Geometry: final body of the model. Coordinates: model frame, mm. Give positions to 0.01 mm unless a question says otherwise; leave off trailing zeros. Write each loop counter-clockwise with the first axis right and the second up, starting at its lowest first coordinate (ties: lowest second). Pieces come first, ordered by that corner, then holes. Notation, with made-up numbers: (43, 88) -> (87, 88) arc R26 ccw to (87, 113) -> close; hole circle Ø9 at (-21, 86.25). An arc over 180 degrees is marked (long way). Answer as a JSON object with one key per item and string values. Group by question number.
(1) Material intervals for probe 1 along Y at (x, z) = (0, 0); probe 2 along X at (y, z) = (0.5, 35); probe 3 along X at (y, z) = (3.5, 13.5), sorted ascending.
(2) Section query A-A on x = 0. Output: boundary loops of the cut face in (y, z), plus the area to 3 significant figures.
(3) Contact query for flat-ended pins moving along their axis: pin 1 Ø8 at (x, z) = (-0.5, 12) entering from -Y; pin 2 Ø13 at (y, z) = (0, 0) entering from -X; pin 3 Ø1.5 at (y, z) = (16, 211.5) entering from +X. Output: stop coordinate, or through.
(4) Section query C-C on z = 237. Output: boundary loops of the cut face in (x, y), plus the area to 3 significant figures.
(5) Section query B-B on y = 0. Output: boundary loops of the cut face in (x, z), plus the area to 3 significant figures.
from build123d import *

# Parameters (mm, degrees)
SKETCH1_R           = 5
BOSS_EXTRUDE1_DEPTH = 5


with BuildPart() as part:
    # Sketch1 → Boss-Extrude1 (new, symmetric)
    with BuildSketch(Plane(origin=(0, 0, 0), x_dir=(0, 0, -1), z_dir=(1, 0, 0))):
        with BuildLine():
            Line((0, -15), (-20, -15))
            Line((-20, -15), (-20, 15))
            Line((-20, 15), (0, 15))
            ThreePointArc((0, 15), (15, 0), (0, -15))
        make_face()
        Circle(SKETCH1_R, mode=Mode.SUBTRACT)
    extrude(amount=BOSS_EXTRUDE1_DEPTH, both=True)

    # Sketch2 → Revolve1 (revolve)
    with BuildSketch(Plane(origin=(0, 0, 0), x_dir=(0, 0, -1), z_dir=(1, 0, 0)), mode=Mode.PRIVATE) as revolve1_sk:
        Polygon((-20, 0), (-20, 20.474587648), (-30.174617149, 20.474587648), (-30.174617149, 17.289208906), (-257.531045689, 17.289208906), (-257.531045689, 11.408509691), (-34.338293907, 11.408509691), (-34.338293907, 0), align=None)
    revolve(revolve1_sk.sketch.rotate(Axis((0, 0, 34.338293907), (0, 0, -1)), 90), axis=Axis((0, 0, 34.338293907), (0, 0, -1)))


solid = part.part
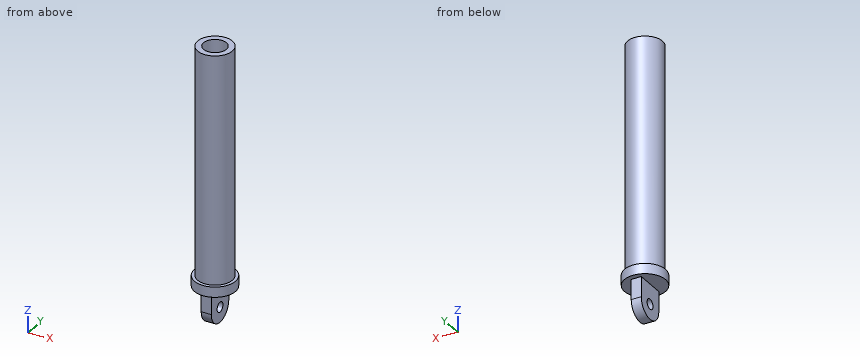
Answer list:
{
 "1": {"probe 1": "-15 to -5, 5 to 15", "probe 2": "-17.28 to -11.4, 11.4 to 17.28", "probe 3": "-5 to 5"},
 "2": {"outline": "(-20.47, 20) -> (-15, 20) -> (-15, 0) arc R15 ccw to (15, 0) -> (15, 20) -> (20.47, 20) -> (20.47, 30.17) -> (17.29, 30.17) -> (17.29, 257.53) -> (11.41, 257.53) -> (11.41, 34.34) -> (-11.41, 34.34) -> (-11.41, 257.53) -> (-17.29, 257.53) -> (-17.29, 30.17) -> (-20.47, 30.17) -> close; hole circle Ø10 at (0, 0)", "area": "4,060 mm2"},
 "3": {"pin 1": "y = -15", "pin 2": "x = -5", "pin 3": "x = 8.15"},
 "4": {"outline": "circle Ø34.58 at (0, 0); hole circle Ø22.82 at (0, 0)", "area": "530 mm2"},
 "5": {"outline": "(-20.47, 20) -> (-5, 20) -> (-5, 5) -> (5, 5) -> (5, 20) -> (20.47, 20) -> (20.47, 30.17) -> (17.29, 30.17) -> (17.29, 257.53) -> (11.41, 257.53) -> (11.41, 34.34) -> (-11.41, 34.34) -> (-11.41, 257.53) -> (-17.29, 257.53) -> (-17.29, 30.17) -> (-20.47, 30.17) -> close; (-5, -15) -> (5, -15) -> (5, -5) -> (-5, -5) -> close", "area": "3,440 mm2"}
}
